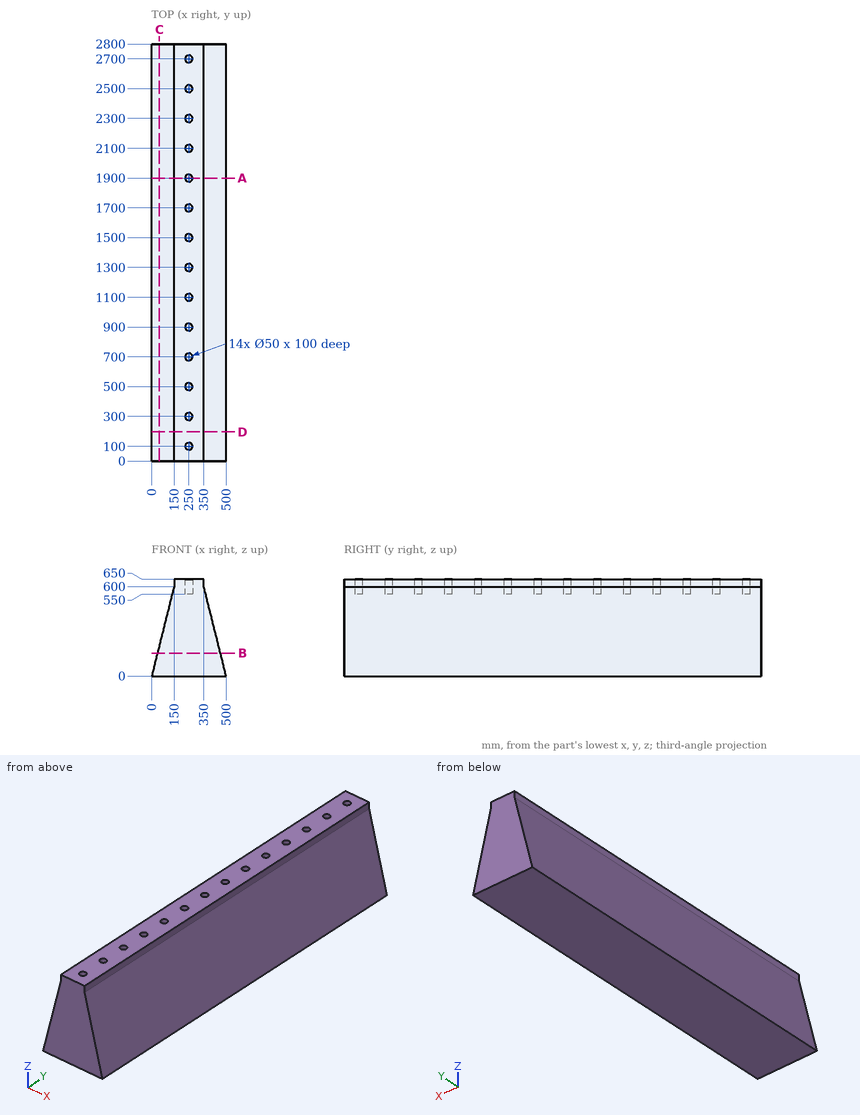
Source: three-view drawing plus pictorial views. Frame: mm from the lowest corner of the part. Coordinates: 2 decimals unless noted, no trailing zeros. Order: outer loops, then holes, each group sorted by start corner. A loop starts at its lowest first (then second) coordinate and runs counter-clockwise, first axis right, second up.
Item 1: Cut plane A-A (y = 1900). Return loops of the section in (x, z).
Output values:
outline: (0, 0) - (500, 0) - (350, 600) - (350, 650) - (275, 650) - (275, 550) - (225, 550) - (225, 650) - (150, 650) - (150, 600) - close
Item 2: First-contact query: P1, Ø15, axis at x = 246.5, y = 711, coming from the +Z side; P2, Ø1, axis at y = 2389.5, z = 483, coming from the -X side (3 decimals); P3, Ø5, axis at y = 1579.5, z = 218.5, coming from the +X side; P4, Ø2, axis at x = 118, z = 311.5, coming from the -Y side. Flat tips, straight axial feed; report the tip coordinate or a pass-through.
Output values:
P1: stops at z = 550
P2: stops at x = 120.625
P3: stops at x = 446
P4: stops at y = 0
Item 3: Cut plane B-B (z = 154). Return loops of the section in (x, y).
Output values:
outline: (38.5, 0) - (461.5, 0) - (461.5, 2800) - (38.5, 2800) - close
Item 4: Cut plane D-D (y = 196). Return loops of the section in (x, z).
Output values:
outline: (0, 0) - (500, 0) - (350, 600) - (350, 650) - (150, 650) - (150, 600) - close
Item 5: Material intervals for line 1 (X direction, y = 1900, z = 624.5); line 2 (X direction, y = 1900, z = 598.5) (3 decimals); line 3 (X direction, y = 1232.5, z = 520), sorted ascending.
Output values:
line 1: x = 150 to 225, 275 to 350
line 2: x = 149.625 to 225, 275 to 350.375
line 3: x = 130 to 370
Item 6: Cut plane C-C (x = 51.5). Return loops of the section in (y, z).
Output values:
outline: (0, 0) - (2800, 0) - (2800, 206) - (0, 206) - close
